```python
from build123d import *

# Parameters (mm, degrees)
ESQUISSE1_W                  = 75
ESQUISSE1_H                  = 70
ESQUISSE1_R                  = 1.5
ESQUISSE1_W_2                = 15
ESQUISSE1_H_2                = 3
BOSS_EXTRU_1_DEPTH           = 3
ENL_V_MAT_EXTRU_1_DEPTH      = 10
ENL_V_MAT_EXTRU_1_DEPTH_BACK = 10


with BuildPart() as part:
    # Esquisse1 → Boss.-Extru.1 (new body)
    with BuildSketch(Plane.XY):
        with Locations((-12.683673469, -2.836734694)):
            Rectangle(ESQUISSE1_W, ESQUISSE1_H)
        with Locations((-38.683673469, 25.663265306)):
            Circle(ESQUISSE1_R, mode=Mode.SUBTRACT)
        with Locations((-38.683673469, 12.663265306)):
            Circle(ESQUISSE1_R, mode=Mode.SUBTRACT)
        with Locations((-38.683673469, -32.836734694)):
            Circle(ESQUISSE1_R, mode=Mode.SUBTRACT)
        with Locations((13.316326531, -32.836734694)):
            Circle(ESQUISSE1_R, mode=Mode.SUBTRACT)
        with Locations((7.316326531, 12.663265306)):
            Rectangle(ESQUISSE1_W_2, ESQUISSE1_H_2, mode=Mode.SUBTRACT)
        with Locations((7.316326531, 25.663265306)):
            Rectangle(ESQUISSE1_W_2, ESQUISSE1_H_2, mode=Mode.SUBTRACT)
    extrude(amount=BOSS_EXTRU_1_DEPTH)

    # Esquisse2 → Enlèv. mat.-Extru.1 (cut, two sides: drawn at the far end of the back side and taken through both)
    with BuildSketch(Plane.XY.offset(-ENL_V_MAT_EXTRU_1_DEPTH_BACK)):
        Polygon((24.816326531, -1.336734694), (18.816326531, -1.336734694), (18.816326531, -0.311734694), (16.766326531, -0.311734694), (16.766326531, -1.336734694), (10.816326531, -1.336734694), (10.816326531, -4.336734694), (16.766326531, -4.336734694), (16.766326531, -5.361734694), (18.816326531, -5.361734694), (18.816326531, -4.336734694), (24.816326531, -4.336734694), align=None)
        Polygon((-50.183673469, -1.336734694), (-50.183673469, -4.336734694), (-44.183673469, -4.336734694), (-44.183673469, -5.361734694), (-42.133673469, -5.361734694), (-42.133673469, -4.336734694), (-36.183673469, -4.336734694), (-36.183673469, -1.336734694), (-42.133673469, -1.336734694), (-42.133673469, -0.311734694), (-44.183673469, -0.311734694), (-44.183673469, -1.336734694), align=None)
    extrude(amount=ENL_V_MAT_EXTRU_1_DEPTH + ENL_V_MAT_EXTRU_1_DEPTH_BACK, mode=Mode.SUBTRACT)


solid = part.part
```
Design review of the part built by this model. Coordinates are the model's own, in mm. A direction names the side the tool comes from. Give positions to 0.01 mm unless a question says otherwise; leave off trailing zeros. Write each loop counter-clockwise with the first axis right and the second up, starting at its lowest first coordinate (ties: lowest second). Pieces come first, ordered by that corner, then holes. Notation, with made-up numbers: (-37.5, 61) - (1.5, 61) arc R22 cw to (1.5, 77) - close; hole circle Ø3 at (2, -4.75). An arc over 180 degrees is marked (long way). Return JSON: item names as keys, results as strings. Group by question number.
(1) Mouldability with a two-part tool opening along X and no side actions: class faces 4 (the cylindrical face through (14.008, -34.167, 1.479)), 5 (the flat face through (10.816, -3, 1)), 6 (the flat face through (14, -1.337, 1)) as +X half, -X half, draft (parallel to the pull), parting line (faces both ways), or undercut.
(2) Machinability: for faces 1 (the flat face through (-47, -4.337, 1)), 2 (the flat face through (7, 14.163, 1)), 3 (the flat face through (-13, -2, 0)), which of the approach directions +Z, -Z, +X, -X, +Y, -Y give a long, thin tool a straight path to every point of the face, cutting with its end or side? Answer none if there is none.
(3) To check wall thickness, follow probe 1 along Y at (x, z) = (9, 1.6); probe 2 along Y at (x, z) = (-41.5, 1.5); probe 3 along Y at (x, z) = (-43.5, 1.95). State the ranges of each line that lie inside material, in increasing order.
(4) We need section A-A, the plane x = 7. Give the boundary of the cut face in (y, z).
(5) We need section B-B, the plane z = 1.35. Give the number of separate pieces and of enclosed holes in the cut face, then the cut area to 3 significant figures.
Reported:
{
 "1": {"face 4": "undercut", "face 5": "+X half", "face 6": "draft"},
 "2": {"face 1": "+Z, -Z, -X", "face 2": "+Z, -Z", "face 3": "-Z, +X, -X, +Y, -Y"},
 "3": {"probe 1": "y = -37.84 to 11.16, 14.16 to 24.16, 27.16 to 32.16", "probe 2": "y = -37.84 to -4.34, -1.34 to 32.16", "probe 3": "y = -37.84 to -5.36, -0.31 to 32.16"},
 "4": {"outline": "(-37.84, 0) - (11.16, 0) - (11.16, 3) - (-37.84, 3) - close; (14.16, 0) - (24.16, 0) - (24.16, 3) - (14.16, 3) - close; (27.16, 0) - (32.16, 0) - (32.16, 3) - (27.16, 3) - close"},
 "5": {"separate pieces": "1", "enclosed holes": "6", "area": "5,040 mm2"}
}
